Check sheet for the modelled part. Datum: model origin and axes. Units: mm. Round coordinates to 2 decimals unless told otherwise and drop trailing zeros. Order: outer loops, then holes, each group sorted by start corner. A loop starts at its lowest first (then second) coordinate and runs counter-clockwise, first axis right, second up. Notation, with made-up numbers: M 42.25,-33.75 L 49.25,-33.75 A15 cw 49.25,-28.75 Z; hole C 60.5,26 d7. An arc over 180 degrees is marked long. One line per item, written item: value. Start each with the question number.
(1) Thickness scan on L1, parallel to Y at x = 0, z = -8; L2, parallel to Y at x = -5, z = 19. Record the ranges inside material, lowest first.
(2) Cross-section at B-B, the plane z = -4. Enter the section's corners in (x, y), and give its area (3 significant figures).
(3) Cross-section at A-A, the plane x = 0. Enter the section's corners in (y, z), and give its area (3 significant figures).
(4) Cross-section at C-C, the plane y = 0. Enter the section's corners in (x, z).
(5) Release check for a two-part mould opening along X. For faces 1 (the face through (6.93, -5.31, -0.43)), 2 (the face through (-42.585, -1, 2)), 3 (the face through (41.057, -100.659, 2.936)) record: released by +X, released by -X, zero draft, split by the parting line, or undercut.
from build123d import *

# Parameters (mm, degrees)
F0_W     = 85.1696208119
F0_H     = 61.5866929293
F1_DEPTH = 102.108
F3_D     = 17.4625
F4_R     = 5.08


with BuildPart() as f1:
    # F0 (on Front) → F1 (new body, symmetric)
    with BuildSketch(Plane.XZ):
        Rectangle(F0_W, F0_H)
    extrude(amount=F1_DEPTH, both=True)

    # F3 (through all)
    with Locations(Plane.XY.offset(30.7933464646)):
        with Locations((0, 0)):
            Hole(F3_D / 2)

    # F4
    f4_edges = [f1.edges().sort_by_distance(p)[0] for p in [
        (0, -102.108, -30.793346),
        (42.58481, 0, -30.793346),
        (0, 102.108, -30.793346),
        (-42.58481, 0, -30.793346),
        (-42.58481, -102.108, 0),
        (-42.58481, 102.108, 0),
        (42.58481, 102.108, 0),
        (42.58481, -102.108, 0),
    ]]
    fillet(f4_edges, radius=F4_R)


solid = f1.part
Values found:
1. L1: -102.11 to -8.73, 8.73 to 102.11
1. L2: -102.11 to -7.16, 7.16 to 102.11
2. outline: M -42.58,-97.03 A5.08 ccw -37.5,-102.11 L 37.5,-102.11 A5.08 ccw 42.58,-97.03 L 42.58,97.03 A5.08 ccw 37.5,102.11 L -37.5,102.11 A5.08 ccw -42.58,97.03 Z; hole C 0,0 d17.46
2. area: 17,100 mm^2
3. outline: M -102.11,-25.71 A5.08 ccw -97.03,-30.79 L -8.73,-30.79 L -8.73,30.79 L -102.11,30.79 Z; M 8.73,-30.79 L 97.03,-30.79 A5.08 ccw 102.11,-25.71 L 102.11,30.79 L 8.73,30.79 Z
3. area: 11,500 mm^2
4. outline: M -42.58,-25.71 A5.08 ccw -37.5,-30.79 L -8.73,-30.79 L -8.73,30.79 L -42.58,30.79 Z; M 8.73,-30.79 L 37.5,-30.79 A5.08 ccw 42.58,-25.71 L 42.58,30.79 L 8.73,30.79 Z
5. face 1: undercut
5. face 2: released by -X
5. face 3: released by +X
